Source: CAD feature listing. Evaluate the final solid. Frame: model axes, mm. Give positions to 0.01 mm unless a question says otherwise; leave off trailing zeros. Loops run counter-clockwise (first coordinate to the right, second up) from the corner with the lowest first, then second, coordinate; pieces in that order, holes last.
from build123d import *

# Parameters (mm, degrees)
PEDOUTLINE_W               = 539.75
PEDOUTLINE_H               = 63.5
PEDOUTLINE_THICKNESS_DEPTH = 17.78
PEDLEDGECUTS_W             = 17.78
PEDLEDGECUTS_H             = 63.5
PEDLEDGECUTS_DEPTH_DEPTH   = 5.08
SKETCH4_R                  = 1.5875
CUT_EXTRUDE2_DEPTH         = 17.78
SKETCH5_R                  = 1.5875
CUT_EXTRUDE3_DEPTH         = 17.78


with BuildPart() as part:
    # PedOutline → PedOutline_Thickness (new body)
    with BuildSketch(Plane.XY):
        with Locations((11108.266666666, -5688.0125)):
            Rectangle(PEDOUTLINE_W, PEDOUTLINE_H)
    extrude(amount=-PEDOUTLINE_THICKNESS_DEPTH)

    # PedLedgeCuts → PedLedgeCuts_Depth (cut)
    with BuildSketch(Plane.XY):
        with Locations((11369.251666666, -5688.0125)):
            Rectangle(PEDLEDGECUTS_W, PEDLEDGECUTS_H)
        with Locations((10847.281666666, -5688.0125)):
            Rectangle(PEDLEDGECUTS_W, PEDLEDGECUTS_H)
    extrude(amount=-PEDLEDGECUTS_DEPTH_DEPTH, mode=Mode.SUBTRACT)

    # Sketch4 → Cut-Extrude2 (cut)
    with BuildSketch(Plane.XY):
        with Locations((10847.281666666, -5668.9625)):
            Circle(SKETCH4_R)
        with Locations((10847.281666666, -5707.0625)):
            Circle(SKETCH4_R)
        with Locations((11369.251666666, -5707.0625)):
            Circle(SKETCH4_R)
        with Locations((11369.251666666, -5668.9625)):
            Circle(SKETCH4_R)
    extrude(amount=-CUT_EXTRUDE2_DEPTH, mode=Mode.SUBTRACT)

    # Sketch5 → Cut-Extrude3 (cut)
    with BuildSketch(Plane(origin=(0, 0, -17.78), x_dir=(-1, 0, 0), z_dir=(0, 0, -1))):
        with Locations((-10911.416666665, -5690.78745)):
            Circle(SKETCH5_R)
        with Locations((-10962.216666665, -5690.78745)):
            Circle(SKETCH5_R)
        with Locations((-11254.316666665, -5690.78745)):
            Circle(SKETCH5_R)
        with Locations((-11305.116666665, -5690.78745)):
            Circle(SKETCH5_R)
    extrude(amount=-CUT_EXTRUDE3_DEPTH, mode=Mode.SUBTRACT)


solid = part.part
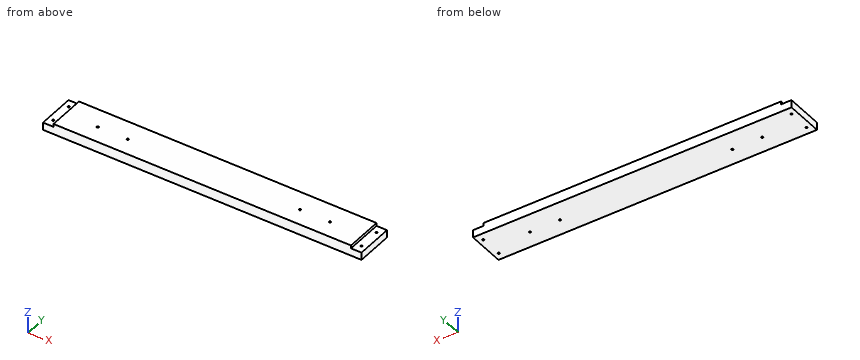
1) Cut plane A-A (y = -5681). Return loops of the section in (x, z).
Checks:
outline: (10838.39, -17.78) - (11378.14, -17.78) - (11378.14, -5.08) - (11360.36, -5.08) - (11360.36, 0) - (10856.17, 0) - (10856.17, -5.08) - (10838.39, -5.08) - close
2) Ray query, probe 1 along X at (y, z) = (-5690.5, -4.75); probe 2 along X at (y, z) = (-5669.5, -8.5); probe 3 along X at (y, z) = (-5690.5, -10.5). Return the intervals inside material, ascending.
Checks:
probe 1: x = 10856.17 to 10909.86, 10912.98 to 10960.66, 10963.78 to 11252.76, 11255.88 to 11303.56, 11306.68 to 11360.36
probe 2: x = 10838.39 to 10845.79, 10848.78 to 11367.76, 11370.75 to 11378.14
probe 3: x = 10838.39 to 10909.86, 10912.98 to 10960.66, 10963.78 to 11252.76, 11255.88 to 11303.56, 11306.68 to 11378.14
3) Contact query for flat-ended pins moving along their axis: P1, Ø1.9, axis at x = 11254.32, y = -5690.79, coming from the -Z side; P2, Ø2.5, axis at y = -5701.5, z = -3, coming from the +X side; P3, Ø4, axis at x = 11305.12, y = -5690.79, coming from the -Z side; P4, Ø4, axis at x = 11369.25, y = -5707.06, coming from the +Z side. Output: stop coordinate, or through.
Checks:
P1: passes through
P2: stops at x = 11360.36
P3: stops at z = -17.78
P4: stops at z = -5.08
